Input: part model. Units: mm. Frame: model coordinates. A direction names the side the tool comes from. Coordinates: 2 decimals unless noted, no trailing zeros. Write each loop counter-clockwise with the first axis right and the second up, starting at its lowest first coordinate (ties: lowest second). Pieces come first, ordered by that corner, then holes. Notation, with made-up numbers: M -18.75,73 L 28.25,73 A17 ccw 28.25,93 Z; hole C 1.25,24.5 d1. An arc over 180 degrees is marked long. Answer as a JSON object with one key per item and string values. Group by question number.
from build123d import *

# Parameters (mm, degrees)
BOSS_EXTRUDE1_DEPTH      = 45.372782
BOSS_EXTRUDE1_DEPTH_BACK = 45.388276
SKETCH1_R                = 32.766
BOSS_EXTRUDE2_DEPTH      = 69.287898
BOSS_EXTRUDE2_DEPTH_BACK = 215.617298
SKETCH2_R                = 38.6334
CUT_EXTRUDE1_DEPTH       = 224.703943753
CUT_EXTRUDE1_DEPTH_BACK  = 224.703943753
SKETCH3_R                = 22.292818
CUT_EXTRUDE2_DEPTH       = 224.703943753
CUT_EXTRUDE2_DEPTH_BACK  = 198.41972
SKETCH4_R                = 29.840301


with BuildPart() as part:
    # Sketch1 → Boss-Extrude1 (new, two sides: drawn at the far end of the back side and taken through both)
    with BuildSketch(Plane(origin=(0, 0, 0), x_dir=(0, 0, -1), z_dir=(1, 0, 0)).offset(-BOSS_EXTRUDE1_DEPTH_BACK)):
        Circle(SKETCH1_R)
    extrude(amount=BOSS_EXTRUDE1_DEPTH + BOSS_EXTRUDE1_DEPTH_BACK)

    # Sketch2 → Boss-Extrude2 (add, two sides: drawn at the far end of the back side and taken through both)
    with BuildSketch(Plane(origin=(0, 0, 0), x_dir=(1, 0, 0), z_dir=(0, 1, 0)).offset(-BOSS_EXTRUDE2_DEPTH_BACK)):
        with Locations(Location((0, 0, 0), (0, 0, 270))):
            Circle(SKETCH2_R)
    extrude(amount=BOSS_EXTRUDE2_DEPTH + BOSS_EXTRUDE2_DEPTH_BACK)

    # Sketch3 → Cut-Extrude1 (cut, two sides: drawn at the far end of the back side and taken through both)
    with BuildSketch(Plane(origin=(0, 0, 0), x_dir=(0, 0, -1), z_dir=(1, 0, 0)).offset(-CUT_EXTRUDE1_DEPTH_BACK)):
        Circle(SKETCH3_R)
    extrude(amount=CUT_EXTRUDE1_DEPTH + CUT_EXTRUDE1_DEPTH_BACK, mode=Mode.SUBTRACT)

    # Sketch4 → Cut-Extrude2 (cut, two sides: drawn at the far end of the back side and taken through both)
    with BuildSketch(Plane(origin=(0, 0, 0), x_dir=(1, 0, 0), z_dir=(0, 1, 0)).offset(-CUT_EXTRUDE2_DEPTH_BACK)):
        with Locations(Location((0, 0, 0), (0, 0, 270))):
            Circle(SKETCH4_R)
    extrude(amount=CUT_EXTRUDE2_DEPTH + CUT_EXTRUDE2_DEPTH_BACK, mode=Mode.SUBTRACT)


solid = part.part
Q1. Pin query (flat end, axial travel): pin 1 Ø3 at (x, z) = (3, -1.5) entering from +Y; pin 2 Ø3 at (x, y) = (16.5, -173.5) entering from +Z; pin 3 Ø3 at (x, y) = (-14.5, -67.5) entering from +Z. Return the tip coordinate at first contact, or that it passes through.
Q2. Section C-C, the plane x = 0. Return the cut outline in (y, z), and give its area (3 significant figures).
Q3. Draft query along Z for faces 1 (the cylindrical face through (-23.508, -75.159, -30.658)), 2 (the flat face through (-45.388, -6.8, -21.4)), 3 (the cylindrical face through (-35.63, -13.565, 17.691)). Return one class per face: released by +Z, released by -Z, zero draft, split by the parting line, or undercut.
Q4. Section D-D, the plane y = -84. Return the cut outline in (x, z).
Q5. Line query: line 1 (X direction, y = -78.5, z = 0); line 2 (Y direction, x = -2, z = -17.5); line 3 (X direction, y = -179, z = -9.5). Output: solid intervals per line, ascending. Write a range as from..to.
Q6. Section B-B, the plane z = 0. Return the cut outline in (x, y), and give its area (3 significant figures).
Q7. Section A-A, the plane y = 0. Return the cut outline in (x, z), and give its area (3 significant figures).
Q8. Access query for faces 4 (the cylindrical face through (38.28, -29.07, -15.12)), 5 (the flat face through (1, -215.617, -1)), 6 (the cylindrical face through (-35.871, 1.441, 32.734)), 7 (the flat face through (0, -198.42, 0)), 8 (the flat face through (45.373, -6.8, -21.4)). Directions: +Z, -Z, +X, -X, +Y, -Y. A direction counts if a zero-diameter tool reaches every point of the face in a straight line with its end or side. Return the directions, or none.
Filled in:
{
 "1": {"pin 1": "y = -198.42", "pin 2": "z = 35.6", "pin 3": "z = 36.38"},
 "2": {"outline": "M -215.62,-38.63 L 69.29,-38.63 L 69.29,-29.84 L -198.42,-29.84 L -198.42,29.84 L 69.29,29.84 L 69.29,38.63 L -215.62,38.63 Z", "area": "6,040 mm^2"},
 "3": {"face 1": "split by the parting line", "face 2": "zero draft", "face 3": "undercut"},
 "4": {"outline": "C 0,0 d77.27; hole C 0,0 d59.68"},
 "5": {"line 1": "-38.63..-29.84, 29.84..38.63", "line 2": "-215.62..-198.42", "line 3": "-37.45..-28.29, 28.29..37.45"},
 "6": {"outline": "M -45.39,-32.77 L -38.63,-32.77 L -38.63,-215.62 L 38.63,-215.62 L 38.63,-32.77 L 45.37,-32.77 L 45.37,-22.29 L 29.84,-22.29 L 29.84,-198.42 L -29.84,-198.42 L -29.84,-22.29 L -45.39,-22.29 Z; M -45.39,22.29 L -29.84,22.29 L -29.84,69.29 L -38.63,69.29 L -38.63,32.77 L -45.39,32.77 Z; M 29.84,22.29 L 45.37,22.29 L 45.37,32.77 L 38.63,32.77 L 38.63,69.29 L 29.84,69.29 Z", "area": "5,540 mm^2"},
 "7": {"outline": "M -45.39,-32.77 L -20.47,-32.77 A38.63 ccw 20.47,-32.77 L 45.37,-32.77 L 45.37,-22.29 L 19.84,-22.29 A29.84 cw -19.84,-22.29 L -45.39,-22.29 Z; M -45.39,22.29 L -19.84,22.29 A29.84 cw 19.84,22.29 L 45.37,22.29 L 45.37,32.77 L 20.47,32.77 A38.63 ccw -20.47,32.77 L -45.39,32.77 Z", "area": "1,820 mm^2"},
 "8": {"face 4": "+X", "face 5": "+Z, -Z, +X, -X, -Y", "face 6": "-X", "face 7": "+Y", "face 8": "+Z, -Z, +X, +Y, -Y"}
}
